Source: CAD feature listing. Evaluate the final solid. Frame: model axes, mm. A direction names the side the tool comes from. Round coordinates to 2 decimals unless told otherwise and drop trailing zeros. Order: outer loops, then holes, each group sorted by start corner. A loop starts at its lowest first (then second) coordinate and runs counter-clockwise, first axis right, second up. Notation, with made-up numbers: M -19,-24 L 20,-24 A7 cw 20,-19 Z; hole C -28,31 d6. An arc over 180 degrees is marked long. Use one line per item in the form item = value. Start each with the question number.
Q1. Contact query for flat-ended pins moving along their axis: pin 1 (2 mm diameter, centred on x = -21, y = 21.5, fed in from -Z); pin 2 (10 mm diameter, centred on y = 52.5, z = 7.5, fed in from -X); pin 3 (7 mm diameter, centred on y = 10, z = 1, fed in from +X). Output: stop coordinate, or through.
Q2. Section B-B (z = 0). Return the cut outline in (x, y) (1 decimal).
Q3. Material intervals for probe 1 along X at (y, z) = (16, 0); probe 2 along Y at (x, z) = (-25, 36) (3 decimals); probe 3 along X at (y, z) = (53.5, 0), sorted ascending.
Q4. Reachability of faces 1 (the flat face through (-43.072, 19, 0)), 2 (the conical face through (31.167, 39.059, 31.777)), 3 (the flat face through (0, 19, -43.072)) from +Z, -Z, +X, -X, +Y, -Y: full face, straight path, thin tool, end or side. Return the list, or none.
Q5. Pull-direction query (Y, two-part tool) for faces 4 (the conical face through (-31.591, 0.174, 30.979)), 5 (the flat face through (-32, 67.945, 17)), 6 (the conical face through (31.777, 39.059, -31.167)); classes: pulls with the +Y half, pulls with the -Y half, needs draft (parallel to the pull), parting line crosses it, or undercut.
Q6. Section A-A (x = 0). Return the cut outline in (y, z) (1 decimal).
Q7. Section C-C (y = 62). Return the cut outline in (x, z).
from build123d import *

# Parameters (mm, degrees)
F0_W            = 67.945
F0_H            = 10.0203
F2_SIZE         = 1
F3_SIZE2        = 1.0208864232
F3_SIZE         = 3.81
F4_W            = 8
F4_H            = 9.8567151233
F7_DEPTH        = 40
F7_COPIES_COUNT = 4
F8_T1_DEPTH     = 46.4577782779
F9_R            = 1
F10_SIZE        = 0.8128
F11_SIZE2       = 2.54
F11_SIZE        = 0.6805909488


# Not quite as in the source:
# - a fillet or chamfer that OpenCascade refuses, or shapes differently, is made with other operations: its cross-section is extruded or revolved along the edge and cut away or added
# - a pattern or mirror of a feature is missing from the dataset's text; its kind, count and spacing are read off the source's solid


with BuildPart() as f1:
    # F0 (on Right) → F1 (revolve)
    with BuildSketch(Plane.YZ):
        with Locations((33.9725, 40.06215)):
            Rectangle(F0_W, F0_H)
    revolve(axis=Axis((0, 10.0695292601, 0), (0, 1, 0)))

    # F2
    f2_edges = [f1.edges().sort_by_distance(p)[0] for p in [
        (0, 0, -35.052),
        (0, 0, -45.0723),
        (0, 67.945, -35.052),
    ]]
    chamfer(f2_edges, length=F2_SIZE)

    # F3
    f3_edges = [f1.edges().sort_by_distance(p)[0] for p in [
        (0, 67.945, -45.0723),
    ]]
    chamfer(f3_edges, length=F3_SIZE, length2=F3_SIZE2)

    # F4 (on Right) → F5 (revolve, cut)
    with BuildSketch(Plane.YZ):
        with Locations((43.5, 46.2033575617)):
            Rectangle(F4_W, F4_H)
    revolve(axis=Axis((0, 33.4974332383, 0), (0, 1, 0)), mode=Mode.SUBTRACT)

    # F6 (on face) → F7 (cut)
    with BuildSketch(Plane.XZ):
        Polygon((3.25, 49.6761292126), (0, 49.6761292126), (-3.25, 49.6761292126), (-3.25, 43.0723), (0, 43.0723), (3.25, 43.0723), align=None)
    f7 = extrude(amount=-F7_DEPTH, mode=Mode.SUBTRACT)

    # F7_copies: F7 ×4 about axis
    f7_copies_axis = Axis((0, 0, 0), (0, 1, 0))
    for i in range(1, F7_COPIES_COUNT):
        add(f7.rotate(f7_copies_axis, i * 360 / F7_COPIES_COUNT), mode=Mode.SUBTRACT)

    # F8: chamfer of 1.5 on 8 edges, made by hand

    # F8_s2 → F8_t1 (cut)
    with BuildSketch(Plane.XZ.offset(-43.478889139)):
        with BuildLine():
            Line((-4.8385212577, 44.8567419714), (-3.2053743546, 43.3889711075))
            Line((-3.2053743546, 43.3889711075), (-3.1753743546, 43.3889711075))
            ThreePointArc((-3.1753743546, 43.3889711075), (-3.22, 44.1719727759), (-3.22, 44.9549744443))
            Line((-3.22, 44.9549744443), (-3.2521631911, 44.9848963528))
            ThreePointArc((-3.2521631911, 44.9848963528), (-4.0455787179, 44.9204937431), (-4.8417120615, 44.8865718016))
            Line((-4.8417120615, 44.8865718016), (-4.8385212577, 44.8567419714))
        make_face()
        with BuildLine():
            Line((4.8385212577, 44.8567419714), (3.2053743546, 43.3889711075))
            Line((3.2053743546, 43.3889711075), (3.1753743546, 43.3889711075))
            ThreePointArc((3.1753743546, 43.3889711075), (3.22, 44.1719727759), (3.22, 44.9549744443))
            Line((3.22, 44.9549744443), (3.2521631911, 44.9848963528))
            ThreePointArc((3.2521631911, 44.9848963528), (4.0455787179, 44.9204937431), (4.8417120615, 44.8865718016))
            Line((4.8417120615, 44.8865718016), (4.8385212577, 44.8567419714))
        make_face()
        with BuildLine():
            Line((-44.8567419714, 4.8385212577), (-43.3889711075, 3.2053743546))
            Line((-43.3889711075, 3.2053743546), (-43.3889711075, 3.1753743546))
            ThreePointArc((-43.3889711075, 3.1753743546), (-44.1719727759, 3.22), (-44.9549744443, 3.22))
            Line((-44.9549744443, 3.22), (-44.9848963528, 3.2521631911))
            ThreePointArc((-44.9848963528, 3.2521631911), (-44.9204937431, 4.0455787179), (-44.8865718016, 4.8417120615))
            Line((-44.8865718016, 4.8417120615), (-44.8567419714, 4.8385212577))
        make_face()
        with BuildLine():
            Line((-43.3889711075, -3.2053743546), (-44.8567419714, -4.8385212577))
            Line((-44.8567419714, -4.8385212577), (-44.8865718016, -4.8417120615))
            ThreePointArc((-44.8865718016, -4.8417120615), (-44.9204937431, -4.0455787179), (-44.9848963528, -3.2521631911))
            Line((-44.9848963528, -3.2521631911), (-44.9549744443, -3.22))
            ThreePointArc((-44.9549744443, -3.22), (-44.1719727759, -3.22), (-43.3889711075, -3.1753743546))
            Line((-43.3889711075, -3.1753743546), (-43.3889711075, -3.2053743546))
        make_face()
        with BuildLine():
            Line((-4.8385212577, -44.8567419714), (-3.2053743546, -43.3889711075))
            Line((-3.2053743546, -43.3889711075), (-3.1753743546, -43.3889711075))
            ThreePointArc((-3.1753743546, -43.3889711075), (-3.22, -44.1719727759), (-3.22, -44.9549744443))
            Line((-3.22, -44.9549744443), (-3.2521631911, -44.9848963528))
            ThreePointArc((-3.2521631911, -44.9848963528), (-4.0455787179, -44.9204937431), (-4.8417120615, -44.8865718016))
            Line((-4.8417120615, -44.8865718016), (-4.8385212577, -44.8567419714))
        make_face()
        with BuildLine():
            Line((3.2053743546, -43.3889711075), (4.8385212577, -44.8567419714))
            Line((4.8385212577, -44.8567419714), (4.8417120615, -44.8865718016))
            ThreePointArc((4.8417120615, -44.8865718016), (4.0455787179, -44.9204937431), (3.2521631911, -44.9848963528))
            Line((3.2521631911, -44.9848963528), (3.22, -44.9549744443))
            ThreePointArc((3.22, -44.9549744443), (3.22, -44.1719727759), (3.1753743546, -43.3889711075))
            Line((3.1753743546, -43.3889711075), (3.2053743546, -43.3889711075))
        make_face()
        with BuildLine():
            Line((44.8567419714, -4.8385212577), (43.3889711075, -3.2053743546))
            Line((43.3889711075, -3.2053743546), (43.3889711075, -3.1753743546))
            ThreePointArc((43.3889711075, -3.1753743546), (44.1719727759, -3.22), (44.9549744443, -3.22))
            Line((44.9549744443, -3.22), (44.9848963528, -3.2521631911))
            ThreePointArc((44.9848963528, -3.2521631911), (44.9204937431, -4.0455787179), (44.8865718016, -4.8417120615))
            Line((44.8865718016, -4.8417120615), (44.8567419714, -4.8385212577))
        make_face()
        with BuildLine():
            Line((43.3889711075, 3.2053743546), (44.8567419714, 4.8385212577))
            Line((44.8567419714, 4.8385212577), (44.8865718016, 4.8417120615))
            ThreePointArc((44.8865718016, 4.8417120615), (44.9204937431, 4.0455787179), (44.9848963528, 3.2521631911))
            Line((44.9848963528, 3.2521631911), (44.9549744443, 3.22))
            ThreePointArc((44.9549744443, 3.22), (44.1719727759, 3.22), (43.3889711075, 3.1753743546))
            Line((43.3889711075, 3.1753743546), (43.3889711075, 3.2053743546))
        make_face()
    extrude(amount=F8_T1_DEPTH, mode=Mode.SUBTRACT)

    # F9
    f9_edges = [f1.edges().sort_by_distance(p)[0] for p in [
        (0, 39.5, -41.275),
        (0, 47.5, -41.275),
    ]]
    fillet(f9_edges, radius=F9_R)

    # F10
    f10_edges = [f1.edges().sort_by_distance(p)[0] for p in [
        (0, 47.5, -45.0723),
    ]]
    chamfer(f10_edges, length=F10_SIZE)

    # F11
    f11_edges = [f1.edges().sort_by_distance(p)[0] for p in [
        (-31.870929, 39.5, 31.870929),
        (-31.870929, 39.5, -31.870929),
        (31.870929, 39.5, -31.870929),
        (31.870929, 39.5, 31.870929),
    ]]
    f11_side = f1.faces().sort_by_distance((0, 39.5, -42.401761))[0]
    chamfer(f11_edges, length=F11_SIZE, length2=F11_SIZE2, reference=f11_side)


solid = f1.part
Results list:
q1.pin_1 = -40.39
q1.pin_2 = -45
q1.pin_3 = 44.55
q2.outline = M -45.1,48.3 L -44.3,47.5 L -42.3,47.5 A1 cw -41.3,46.5 L -41.3,40.5 A1 cw -42.3,39.5 L -43.1,39.5 L -43.1,0 L -36.1,0 L -35.1,1 L -35.1,66.9 L -36.1,67.9 L -44.1,67.9 L -45.1,64.1 Z; M 35.1,1 L 36.1,0 L 43.1,0 L 43.1,39.5 L 42.3,39.5 A1 cw 41.3,40.5 L 41.3,46.5 A1 cw 42.3,47.5 L 44.3,47.5 L 45.1,48.3 L 45.1,64.1 L 44.1,67.9 L 36.1,67.9 L 35.1,66.9 Z
q3.probe_1 = -43.07 to -35.05, 35.05 to 43.07
q3.probe_2 = 0 to 39.5, 47.5 to 67.945
q3.probe_3 = -45.07 to -35.05, 35.05 to 45.07
q4.face_1 = -X, -Y
q4.face_2 = +Z, +X
q4.face_3 = -Z, -Y
q5.face_4 = pulls with the -Y half
q5.face_5 = pulls with the +Y half
q5.face_6 = undercut
q6.outline = M 0,-43.1 L 39.5,-43.1 L 39.5,-42.3 A1 cw 40.5,-41.3 L 46.5,-41.3 A1 cw 47.5,-42.3 L 47.5,-44.3 L 48.3,-45.1 L 64.1,-45.1 L 67.9,-44.1 L 67.9,-36.1 L 66.9,-35.1 L 1,-35.1 L 0,-36.1 Z; M 0,36.1 L 1,35.1 L 66.9,35.1 L 67.9,36.1 L 67.9,44.1 L 64.1,45.1 L 48.3,45.1 L 47.5,44.3 L 47.5,42.3 A1 cw 46.5,41.3 L 40.5,41.3 A1 cw 39.5,42.3 L 39.5,43.1 L 0,43.1 Z
q7.outline = C 0,0 d90.14; hole C 0,0 d70.1
